Design review of the part built by this model. Coordinates are the model's own, in mm. Face numbers are marked on the shaded views. Round coordinates to 2 decimals unless told otherwise and drop trailing zeros. Order: outer loops, then holes, each group sorted by start corner. A loop starts at its lowest first (then second) coordinate and runs counter-clockwise, first axis right, second up. Notation, with made-up numbers: (-10.75, 29.25) - (47.25, 29.25) arc R11 cw to (47.25, 34.25) - close; hole circle Ø7 at (67, 12). An arc over 180 degrees is marked (long way). Write item = value, one per line.
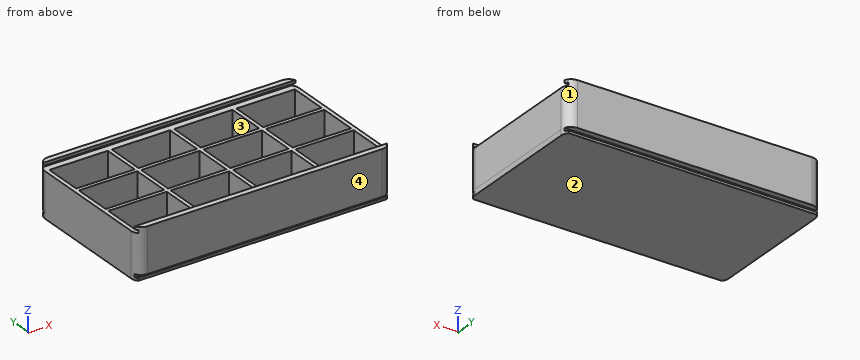
from build123d import *

# Parameters (mm, degrees)
CROQUIS1_W           = 130.242640688
CROQUIS1_H           = 68.242640688
CROQUIS1_W_2         = 30
CROQUIS1_H_2         = 20
CELDAS_DEPTH         = 20
BASE_START           = -128.12132
CROQUIS2_W           = 2
CROQUIS2_H           = 68.242640688
BASE_DEPTH           = 126
EXCEDENTE_DEPTH      = 3
EXCEDENTE_DEPTH_BACK = 20
CROQUIS3_W           = 130.242640688
CROQUIS3_H           = 3
CROQUIS4_W           = 1.5
CROQUIS4_H           = 71.242640688
RANURA_DEPTH         = 150.231036917
PESTA_A_DEPTH        = 130.242641
F_3D_FIX_DEPTH       = 150.23103719
REDONDEO_R           = 5


with BuildPart() as part:
    # Croquis1 → Celdas (new body)
    with BuildSketch(Plane.XY):
        with Locations((63, -32)):
            Rectangle(CROQUIS1_W, CROQUIS1_H)
        with Locations((47, -10)):
            Rectangle(CROQUIS1_W_2, CROQUIS1_H_2, mode=Mode.SUBTRACT)
        with Locations((15, -10)):
            Rectangle(CROQUIS1_W_2, CROQUIS1_H_2, mode=Mode.SUBTRACT)
        with Locations((79, -10)):
            Rectangle(CROQUIS1_W_2, CROQUIS1_H_2, mode=Mode.SUBTRACT)
        with Locations((111, -10)):
            Rectangle(CROQUIS1_W_2, CROQUIS1_H_2, mode=Mode.SUBTRACT)
        with Locations((47, -32)):
            Rectangle(CROQUIS1_W_2, CROQUIS1_H_2, mode=Mode.SUBTRACT)
        with Locations((79, -32)):
            Rectangle(CROQUIS1_W_2, CROQUIS1_H_2, mode=Mode.SUBTRACT)
        with Locations((111, -32)):
            Rectangle(CROQUIS1_W_2, CROQUIS1_H_2, mode=Mode.SUBTRACT)
        with Locations((47, -54)):
            Rectangle(CROQUIS1_W_2, CROQUIS1_H_2, mode=Mode.SUBTRACT)
        with Locations((79, -54)):
            Rectangle(CROQUIS1_W_2, CROQUIS1_H_2, mode=Mode.SUBTRACT)
        with Locations((111, -54)):
            Rectangle(CROQUIS1_W_2, CROQUIS1_H_2, mode=Mode.SUBTRACT)
        with Locations((15, -32)):
            Rectangle(CROQUIS1_W_2, CROQUIS1_H_2, mode=Mode.SUBTRACT)
        with Locations((15, -54)):
            Rectangle(CROQUIS1_W_2, CROQUIS1_H_2, mode=Mode.SUBTRACT)
    extrude(amount=CELDAS_DEPTH)


with BuildPart() as base_tool:
    # Croquis2 → Base (new body)
    with BuildSketch(Plane(origin=(128.121320344, 0, 0), x_dir=(0, 0, -1), z_dir=(1, 0, 0)).offset(BASE_START)):
        with Locations((-1, -32)):
            Rectangle(CROQUIS2_W, CROQUIS2_H)
    extrude(amount=BASE_DEPTH)


with BuildPart() as part_1:
    add(part.part)


with BuildPart() as part_2:
    # Base: joined with base_tool
    add(part_1.part.fuse(base_tool.part, tol=0.00001))

    # Croquis3 → Excedente (add, two sides: drawn at the far end of the back side and taken through both)
    with BuildSketch(Plane.XY.offset(20).offset(-EXCEDENTE_DEPTH_BACK)):
        with Locations((63, -67.621320344)):
            Rectangle(CROQUIS3_W, CROQUIS3_H)
        with Locations((63, 3.621320344)):
            Rectangle(CROQUIS3_W, CROQUIS3_H)
    extrude(amount=EXCEDENTE_DEPTH + EXCEDENTE_DEPTH_BACK)

    # Croquis4 → Ranura (cut, through all)
    with BuildSketch(Plane.ZY.offset(2.121320344)):
        with Locations((20.75, -32)):
            Rectangle(CROQUIS4_W, CROQUIS4_H)
    extrude(amount=-RANURA_DEPTH, mode=Mode.SUBTRACT)

    # Croquis6 → Pestaña (add, through all)
    with BuildSketch(Plane.ZY.offset(2.121320344)):
        Polygon((0, 2.121320344), (0, -66.121320344), (-1.5, -66.121320344), (-1.5, -67.621320344), (-3, -67.621320344), (-3, 3.621320344), (-1.5, 3.621320344), (-1.5, 2.121320344), align=None)
    extrude(amount=-PESTA_A_DEPTH)

    # Croquis7 → 3D-Fix (cut, through all)
    with BuildSketch(Plane.ZY.offset(2.121320344)):
        Polygon((-0.1, 2.021320344), (-1.6, 2.021320344), (-1.6, 3.521320344), (-2.9, 3.521320344), (-2.9, -67.521320344), (-1.6, -67.521320344), (-1.6, -66.021320344), (-0.1, -66.021320344), (0, -66.021320344), (0, -66.121320344), (-1.5, -66.121320344), (-1.5, -67.621320344), (-3, -67.621320344), (-3, 3.621320344), (-1.5, 3.621320344), (-1.5, 2.121320344), (0, 2.121320344), (0, 2.021320344), align=None)
    extrude(amount=-F_3D_FIX_DEPTH, mode=Mode.SUBTRACT)

    # Redondeo
    # the kernel refuses this fillet: 5 mm, written as the material it takes off along each edge
    with BuildSketch(Plane(origin=(128.121320344, 5.121320344, -12.5), x_dir=(0, -1, 0), z_dir=(0, 0, 1)), Plane(origin=(128.121320344, -69.121320344, 35.5), x_dir=(0, 1, 0), z_dir=(0, 0, -1)), Plane(origin=(-2.121320344, -69.121320344, -12.5), x_dir=(0, 1, 0), z_dir=(0, 0, 1))) as redondeo_piece_1:
        with BuildLine():
            CenterArc((REDONDEO_R, -REDONDEO_R), REDONDEO_R, 90, 90)
            Line((0, -REDONDEO_R), (0, 0))
            Line((0, 0), (REDONDEO_R, 0))
        make_face()
    extrude(amount=48, mode=Mode.SUBTRACT)
    with BuildSketch(Plane(origin=(-2.121320344, 5.121320344, 35.5), x_dir=(1, 0, 0), z_dir=(0, 0, -1))) as redondeo_piece_2:
        with BuildLine():
            CenterArc((REDONDEO_R, REDONDEO_R), REDONDEO_R, 180, 90)
            Line((0, REDONDEO_R), (0, 0))
            Line((0, 0), (REDONDEO_R, 0))
        make_face()
    extrude(amount=48, mode=Mode.SUBTRACT)


solid = part_2.part
1) We need section C-C on z = 3.25. Give the number of separate pieces and of enclosed holes in the cut face, and give its area (3 significant figures).
Findings:
separate_pieces = 1
enclosed_holes = 12
area = 2,450 mm^2
2) We need section A-A on y = -14.5. Write out the cut boundary in (x, z).
Findings:
outline = (-2.12, -2.9) - (128.12, -2.9) - (128.12, 20) - (126, 20) - (126, 2) - (96, 2) - (96, 20) - (94, 20) - (94, 2) - (64, 2) - (64, 20) - (62, 20) - (62, 2) - (32, 2) - (32, 20) - (30, 20) - (30, 2) - (0, 2) - (0, 20) - (-2.12, 20) - close
3) Clearance check with flat-ended pins moving along their axes: pin 1 Ø10 at (x, y) = (116.5, -36.5) entering from +Z; pin 2 Ø8 at (x, y) = (75.5, -61.5) entering from +Z. State where each tip first meets the part, or that it passes through.
Findings:
pin_1 = 2
pin_2 = 20
4) The part is to be moulded in two halves that separate along Y. For the marked faces 1, 2, 3 and 4, say which applies: released by +Y, released by -Y, zero draft, split by the parting line, or undercut.
Findings:
face_1 = released by +Y
face_2 = zero draft
face_3 = undercut
face_4 = released by -Y
5) To check wall thickness, follow L1, parallel to X at y = -48.5, z = 10.75; L2, parallel to Y at x = 35, z = 11; L3, parallel to Y at x = 119, z = 21. State the ranges of each line that lie inside material, in increasing order. Write a range as from..to.
Findings:
L1 = -2.12..0, 30..32, 62..64, 94..96, 126..128.12
L2 = -69.12..-64, -44..-42, -22..-20, 0..5.12
L3 = -69.12..-67.62, 3.62..5.12
